Can you work these out from the model? Positions are in its coordinate system, mm. Face numbers are marked on the shaded views. A direction names the side the tool comes from. Give positions to 0.01 mm unless a question says otherwise; leave off trailing zeros. Order: outer loops, then holes, each group sorted by start corner. A loop starts at its lowest first (then second) coordinate and runs counter-clockwise, first axis right, second up.
Item 1: I want a section at A-A, the plane z = -4.75. Write out the boundary of the cut face in (x, y).
Item 2: If we mould it in two halves opening along Y, with no side actions, what happens to the marked faces 4, 5 and 6? For each: +Y half, -Y half, draft (parallel to the pull), parting line (faces both ways), or undercut.
Item 3: I'm going to push flat-ended pins straight in: pin 1 Ø1 at (y, z) = (0, -0.5) entering from +X; pin 2 Ø1.5 at (x, y) = (0, 0) entering from +Z; pin 3 Ø1.5 at (x, z) = (3, -6) entering from +Y; pin 4 Ø1 at (x, z) = (-3.5, -4.5) entering from +Y. Where does each tip first touch, or does it pass through?
Item 4: Which directions (+Z, -Z, +X, -X, +Y, -Y) give clear straight access to the entire face, cutting with the end or side of a thin tool? Please do the marked faces 1, 2 and 3.
Item 5: If I drill on line 1 along Y through (x, z) = (-5.6, 0); line 2 along X through (y, z) = (0.7, 4); line 3 along Z through (x, y) = (-4, 1.1) (3 decimals), over which ranges is the centre line in solid material (lowest first)?
Autodesk Inventor part; units mm, degrees
ref_plane "YZ Plane" through (0, 0, 0) normal (1, 0, 0) x (0, 1, 0)
ref_plane "XZ Plane" through (0, 0, 0) normal (0, 1, 0) x (-1, 0, 0)
ref_plane "XY Plane" through (0, 0, 0) normal (0, 0, 1) x (1, 0, 0)
sketch "Sketch1" plane through (0, 0, 0) normal (0, 0, 1) x (1, 0, 0)
  circle A0 centre (0, 0) radius 2.5
  dimension "d0" = 5
extrude "Extrusion1" add sketch "Sketch1" along normal mid plane 16.1
sketch "Sketch2" plane through (0, 0, 8.05) normal (0, 0, 1) x (1, 0, 0)
  circle A0 centre (0, 0) radius 1.25
  dimension "d3" = 2.5
extrude "Extrusion2" cut sketch "Sketch2" against normal blind 0.25
mirror "Mirror1" about plane through (0, 0, 0) normal (0, 0, 1) of "Extrusion2"
sketch "Sketch3" plane through (0, 0, 0) normal (1, 0, 0) x (0, 1, 0)
  circle A0 centre (0, 0) radius 2.5
  dimension "d6" = 5
extrude "Extrusion3" add sketch "Sketch3" along normal mid plane 11.6
sketch "Sketch4" plane through (5.8, 0, 0) normal (1, 0, 0) x (0, 0, -1)
  circle A0 centre (0, 0) radius 1.25
  dimension "d9" = 2.5
extrude "Extrusion4" cut sketch "Sketch4" against normal blind 0.35
mirror "Mirror2" about plane through (0, 0, 0) normal (1, 0, 0) of "Extrusion4"
fillet "Fillet1" radius 1.5 6 edges at (1.7678, 1.7678, 1.7678) (-2.5, 0, 2.5) (1.7678, -1.7678, 1.7678) (1.7678, -1.7678, -1.7678) (1.7678, 1.7678, -1.7678) (-2.5, 0, -2.5)
ref_plane "Work Plane1" through (0, 0, 0) normal (1, 0, 0) x (0, 1, 0)
properties part number "Cross_Normal"
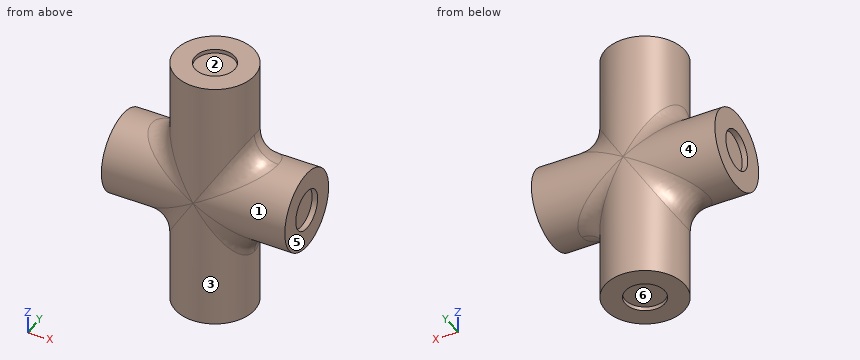
Results list:
1. outline: circle Ø5 at (0, 0)
2. face 4: parting line
2. face 5: draft
2. face 6: undercut
3. pin 1: stops at x = 5.45
3. pin 2: stops at z = 7.8
3. pin 3: stops at y = 1.09
3. pin 4: passes through
4. face 1: +X
4. face 2: +Z
4. face 3: -Z
5. line 1: y = -2.5 to -1.25, 1.25 to 2.5
5. line 2: x = -2.4 to 2.4
5. line 3: z = -2.245 to 2.245
